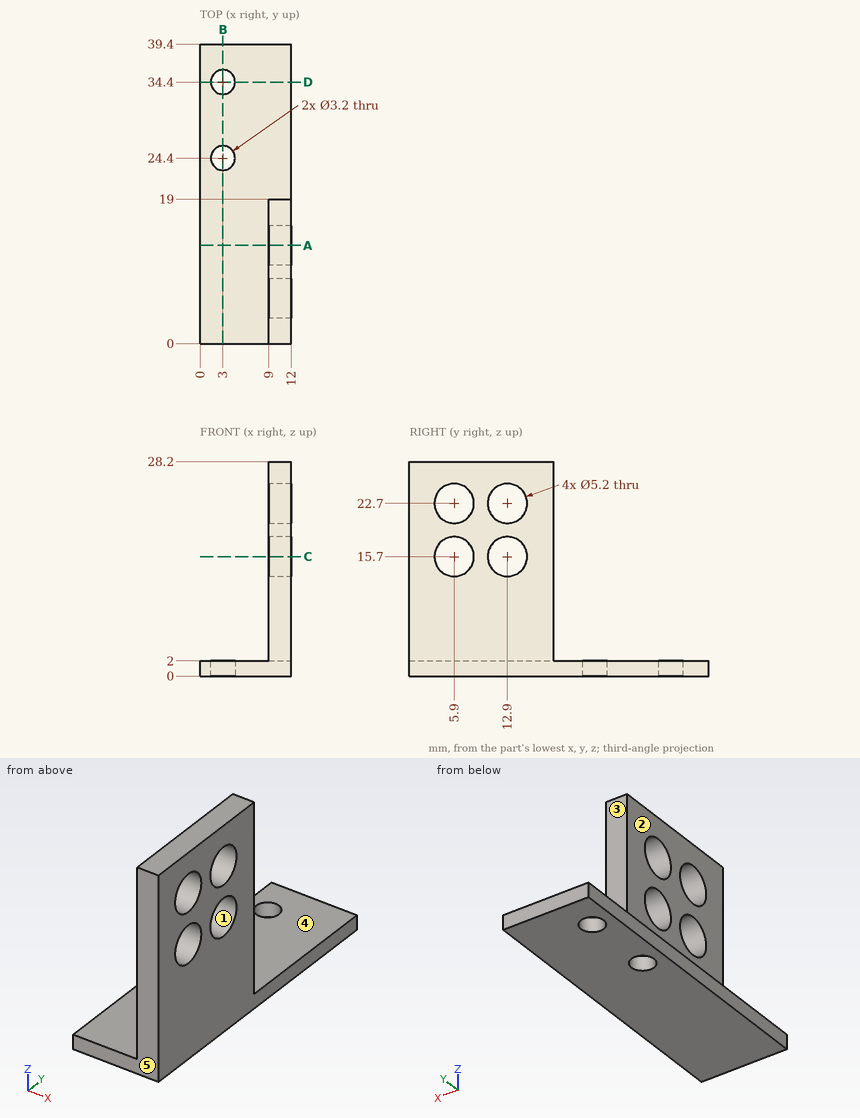
Design review of the part shown in the three views and the two pictorial views. Dimensions are in mm from the part's minimum x, y and z. A direction names the side the tool comes from. Give positions to 0.01 mm unless a question says otherwise; leave off trailing zeros. Loops run counter-clockwise (first coordinate to the right, second up) from the corner with the lowest first, then second, coordinate; pieces in that order, holes last. Notation, with made-up numbers: (50, 15.25) -> (71, 15.25) arc R10 cw to (71, 22.25) -> close; hole circle Ø7 at (-29, 62). An arc over 180 degrees is marked (long way). Put each result on its own line as item: value. Start each with the question number.
1. Clearance check with flat-ended pins moving along their axes: P1, Ø3, axis at x = 10, z = 6, coming from the -Y side; P2, Ø1.5, axis at x = 4, y = 29.5, coming from the +Z side; P3, Ø9.5, axis at y = 12, z = 13.5, coming from the -X side; P4, Ø2.5, axis at x = 10.5, z = 20, coming from the +Y side. State where each tip first meets the part, or that it passes through.
2. Mouldability with a two-part tool opening along Y and no side actions: class the marked faces 1, 2 and 3 as released by +Y, released by -Y, zero draft, split by the parting line, or undercut.
3. We need section D-D on y = 34.4. State the section outline as (x, z) points.
4. We need section C-C on z = 15.7. State the section outline as (x, y) points, then the cut area to 3 significant figures.
5. We need section A-A on y = 12.9. State the section outline as (x, z) points, then the cut area to 3 significant figures.
6. Wall thickness on probe 1 along Z at (x, y) = (11.2, 5.9); probe 2 along Y at (x, z) = (9.9, 15.7); probe 3 along Y at (x, z) = (3, 0.7): over which ranges is each line inside the solid? List them lowest first.
7. For the marked faces 4 and 5, list the 3-axis set-ups (+Z, -Z, +X, -X, +Y, -Y) from which the entire face can be reached by the end or side of a thin tool; tool diameter is ignored.
8. We need section B-B on x = 3. State the section outline as (y, z) points.
Determined:
1. P1: y = 0
1. P2: z = 2
1. P3: x = 9
1. P4: y = 19
2. face 1: undercut
2. face 2: zero draft
2. face 3: released by +Y
3. outline: (0, 0) -> (1.4, 0) -> (1.4, 2) -> (0, 2) -> close; (4.6, 0) -> (12, 0) -> (12, 2) -> (4.6, 2) -> close
4. outline: (9, 0) -> (12, 0) -> (12, 3.3) -> (9, 3.3) -> close; (9, 8.5) -> (12, 8.5) -> (12, 10.3) -> (9, 10.3) -> close; (9, 15.5) -> (12, 15.5) -> (12, 19) -> (9, 19) -> close
4. area: 25.8 mm^2
5. outline: (0, 0) -> (12, 0) -> (12, 13.1) -> (9, 13.1) -> (9, 2) -> (0, 2) -> close; (9, 18.3) -> (12, 18.3) -> (12, 20.1) -> (9, 20.1) -> close; (9, 25.3) -> (12, 25.3) -> (12, 28.2) -> (9, 28.2) -> close
5. area: 71.4 mm^2
6. probe 1: 0 to 13.1, 18.3 to 20.1, 25.3 to 28.2
6. probe 2: 0 to 3.3, 8.5 to 10.3, 15.5 to 19
6. probe 3: 0 to 22.8, 26 to 32.8, 36 to 39.4
7. face 4: +Z, -X, +Y
7. face 5: +Z, -Z, +X, -X, -Y
8. outline: (0, 0) -> (22.8, 0) -> (22.8, 2) -> (0, 2) -> close; (26, 0) -> (32.8, 0) -> (32.8, 2) -> (26, 2) -> close; (36, 0) -> (39.4, 0) -> (39.4, 2) -> (36, 2) -> close
